The model under review builds one solid part; all positions refer to its coordinate system, in mm. A direction names the side the tool comes from. Give positions to 0.01 mm unless a question says otherwise; leave off trailing zeros. Loops run counter-clockwise (first coordinate to the right, second up) from the corner with the lowest first, then second, coordinate; pieces in that order, holes last. Notation, with made-up numbers: (-13, 71.5) - (24, 71.5) arc R26 ccw to (24, 87.5) - close; hole circle Ø5 at (-26, 57). An arc over 180 degrees is marked (long way). Return JSON: item names as keys, results as strings. Group by question number.
```python
from build123d import *

# Parameters (mm, degrees)
BOSS_EXTRUDE1_DEPTH = 24
SKETCH3_R           = 1.1
BOSS_EXTRUDE6_DEPTH = 2
SHELL1_START        = 2.5
SHELL1_OUTLINE_W    = 40
SHELL1_OUTLINE_H    = 21
SHELL1_DEPTH        = 10.5
SHELL1_START_2      = 12.5
SHELL1_2_DEPTH      = 0.5
SHELL1_START_3      = 1.5
SHELL1_3_DEPTH      = 21
CUT_EXTRUDE1_START  = 16.6
SKETCH5_W           = 3.5
SKETCH5_H           = 5
CUT_EXTRUDE1_DEPTH  = 4.9
FILLET1_R           = 0.5


with BuildPart() as part:
    # Sketch1 → Boss-Extrude1 (new body)
    with BuildSketch(Plane.XY):
        with BuildLine():
            Line((-21.5, 13), (21.5, 13))
            Line((21.5, 13), (21.5, 2.5))
            ThreePointArc((21.5, 2.5), (20.767766953, 0.732233047), (19, 0))
            Line((19, 0), (-19, 0))
            ThreePointArc((-19, 0), (-20.767766953, 0.732233047), (-21.5, 2.5))
            Line((-21.5, 2.5), (-21.5, 13))
        make_face()
    extrude(amount=BOSS_EXTRUDE1_DEPTH)

    # Sketch3 → Boss-Extrude6 (add)
    # profile 1 of 4: a face of its own
    with BuildSketch(Plane(origin=(0, 13, 0), x_dir=(-1, 0, 0), z_dir=(0, 1, 0))):
        with BuildLine():
            Line((16.6, 0), (10.4, 0))
            Line((10.4, 0), (10.4, -2.5))
            ThreePointArc((10.4, -2.5), (13.5, -5.6), (16.6, -2.5))
            Line((16.6, -2.5), (16.6, 0))
        make_face()
        with Locations(Location((13.5, -2.5, 0), (0, 0, 90))):
            Circle(SKETCH3_R, mode=Mode.SUBTRACT)
    # profile 2 of 4: a face of its own
    with BuildSketch(Plane(origin=(0, 13, 0), x_dir=(-1, 0, 0), z_dir=(0, 1, 0))):
        with BuildLine():
            Line((-10.4, 0), (-16.6, 0))
            Line((-16.6, 0), (-16.6, -2.5))
            ThreePointArc((-16.6, -2.5), (-13.5, -5.6), (-10.4, -2.5))
            Line((-10.4, -2.5), (-10.4, 0))
        make_face()
        with Locations(Location((-13.5, -2.5, 0), (0, 0, 90))):
            Circle(SKETCH3_R, mode=Mode.SUBTRACT)
    # profile 3 of 4: a face of its own
    with BuildSketch(Plane(origin=(0, 13, 0), x_dir=(-1, 0, 0), z_dir=(0, 1, 0))):
        with BuildLine():
            Line((-16.6, 26.5), (-16.6, 24))
            Line((-16.6, 24), (-10.4, 24))
            Line((-10.4, 24), (-10.4, 26.5))
            ThreePointArc((-10.4, 26.5), (-13.5, 29.6), (-16.6, 26.5))
        make_face()
        with Locations(Location((-13.5, 26.5, 0), (0, 0, 90))):
            Circle(SKETCH3_R, mode=Mode.SUBTRACT)
    # profile 4 of 4: a face of its own
    with BuildSketch(Plane(origin=(0, 13, 0), x_dir=(-1, 0, 0), z_dir=(0, 1, 0))):
        with BuildLine():
            Line((10.4, 26.5), (10.4, 24))
            Line((10.4, 24), (16.6, 24))
            Line((16.6, 24), (16.6, 26.5))
            ThreePointArc((16.6, 26.5), (13.5, 29.6), (10.4, 26.5))
        make_face()
        with Locations(Location((13.5, 26.5, 0), (0, 0, 90))):
            Circle(SKETCH3_R, mode=Mode.SUBTRACT)
    extrude(amount=-BOSS_EXTRUDE6_DEPTH)

    # Shell1: read off the stored shape, not the designer's step
    # Shell1 outline → Shell1 (cut)
    with BuildSketch(Plane(origin=(0, 0, 0), x_dir=(1, 0, 0), z_dir=(0, 1, 0)).offset(SHELL1_START)):
        with Locations((0, -12)):
            Rectangle(SHELL1_OUTLINE_W, SHELL1_OUTLINE_H)
    extrude(amount=SHELL1_DEPTH, mode=Mode.SUBTRACT)

    # Shell1 2 outline → Shell1 2 (cut)
    with BuildSketch(Plane(origin=(0, 0, 0), x_dir=(1, 0, 0), z_dir=(0, 1, 0)).offset(SHELL1_START_2)):
        with BuildLine():
            Line((-15.1, 0.450609847), (-15.1, -1.5))
            Line((-15.1, -1.5), (-11.9, -1.5))
            Line((-11.9, -1.5), (-11.9, 0.450609847))
            ThreePointArc((-11.9, 0.450609847), (-13.5, -0.1), (-15.1, 0.450609847))
        make_face()
        with BuildLine():
            Line((-11.9, -22.5), (-15.1, -22.5))
            Line((-15.1, -22.5), (-15.1, -24.450609847))
            ThreePointArc((-15.1, -24.450609847), (-13.5, -23.9), (-11.9, -24.450609847))
            Line((-11.9, -24.450609847), (-11.9, -22.5))
        make_face()
        with BuildLine():
            Line((11.9, 0.450609847), (11.9, -1.5))
            Line((11.9, -1.5), (15.1, -1.5))
            Line((15.1, -1.5), (15.1, 0.450609847))
            ThreePointArc((15.1, 0.450609847), (13.5, -0.1), (11.9, 0.450609847))
        make_face()
        with BuildLine():
            Line((15.1, -22.5), (11.9, -22.5))
            Line((11.9, -22.5), (11.9, -24.450609847))
            ThreePointArc((11.9, -24.450609847), (13.5, -23.9), (15.1, -24.450609847))
            Line((15.1, -24.450609847), (15.1, -22.5))
        make_face()
    extrude(amount=SHELL1_2_DEPTH, mode=Mode.SUBTRACT)

    # Shell1 3 outline → Shell1 3 (cut)
    with BuildSketch(Plane.XY.offset(SHELL1_START_3)):
        with BuildLine():
            ThreePointArc((19, 1.5), (19.707106781, 1.792893219), (20, 2.5))
            Line((20, 2.5), (-20, 2.5))
            ThreePointArc((-20, 2.5), (-19.707106781, 1.792893219), (-19, 1.5))
            Line((-19, 1.5), (19, 1.5))
        make_face()
    extrude(amount=SHELL1_3_DEPTH, mode=Mode.SUBTRACT)

    # Sketch5 → Cut-Extrude1 (cut)
    with BuildSketch(Plane(origin=(0, 0, 0), x_dir=(0, 0, -1), z_dir=(1, 0, 0)).offset(CUT_EXTRUDE1_START)):
        with Locations((-22.25, 10.5)):
            Rectangle(SKETCH5_W, SKETCH5_H)
    extrude(amount=CUT_EXTRUDE1_DEPTH, mode=Mode.SUBTRACT)

    # Fillet1
    fillet1_edges = [part.edges().sort_by_distance(p)[0] for p in [
        (-10.4, 12, 24),
        (-16.6, 12, 24),
        (10.4, 12, 24),
        (10.4, 12, 0),
        (16.6, 12, 0),
        (-10.4, 12, 0),
        (-16.6, 12, 0),
        (13.5, 11, 0),
        (-13.5, 11, 0),
        (13.5, 11, 24),
        (-13.5, 11, 24),
    ]]
    fillet(fillet1_edges, radius=FILLET1_R)


solid = part.part
```
1) Tool access review of faces 1 (the face through (-14, 11, -4)), 2 (the face through (-20, 8, 12)), 3 (the face through (10.4, 12, 25)), 4 (the face through (-16.6, 12, -2)): name each direction out of +Z, -Z, +X, -X, +Y, -Y from which nothing blocks a thin tool from reaching the whole face with its end or side.
2) For pin 1 Ø1 at (y, z) = (12.5, 25.5) entering from -X; pin 2 Ø0.6 at (x, z) = (13, 23.5) entering from +Y; pin 3 Ø3 at (x, y) = (-4, 7.5) entering from +Z, all flat-tipped, find the tip position at first contact; note any pin that passes through.
3) We need section C-C, the plane z = 5.5. Write out the cut boundary in (x, y), plus the area to 3 significant figures.
4) Draft analysis for pull direction Z (two halves, no side actions). For faces 5 (the face through (13, 12.5, 23)), 6 (the face through (-10.4, 12, 26)), 7 (the face through (13.6, 12, -5.6)), 8 (the face through (13.4, 12, 29.6)), state which applies: +Z half, -Z half, draft (parallel to the pull), parting line (faces both ways), or undercut.
5) We need section A-A, the plane y = 4.25. Write out the cut boundary in (x, z).
6) We need section B-B, the plane x = -13.5. Write out the cut boundary in (y, z).
7) To check wall thickness, follow line 1 (X direction, y = 12.5, z = 26.5); line 2 (Z direction, x = 0, y = 10.5); line 3 (X direction, y = 11.25, z = 8). State the ranges of each line that lie inside material, in increasing order.
8) We need section D-D, the plane x = -4. Write out the cut boundary in (y, z), plus the area to 3 significant figures.
Findings:
{
 "1": {"face 1": "-Z, +X, -X, -Y", "face 2": "+Y", "face 3": "+Z, +Y, -Y", "face 4": "-Z, -X, +Y, -Y"},
 "2": {"pin 1": "stops at x = -16.6", "pin 2": "stops at y = 12.5", "pin 3": "stops at z = 24"},
 "3": {"outline": "(-21.5, 2.5) arc R2.5 ccw to (-19, 0) - (19, 0) arc R2.5 ccw to (21.5, 2.5) - (21.5, 13) - (20, 13) - (20, 2.5) arc R1 cw to (19, 1.5) - (-19, 1.5) arc R1 cw to (-20, 2.5) - (-20, 13) - (-21.5, 13) - close", "area": "96.7 mm^2"},
 "4": {"face 5": "undercut", "face 6": "draft", "face 7": "-Z half", "face 8": "+Z half"},
 "5": {"outline": "(-21.5, 0) - (21.5, 0) - (21.5, 24) - (-21.5, 24) - close; hole (-20, 1.5) - (20, 1.5) - (20, 22.5) - (-20, 22.5) - close"},
 "6": {"outline": "(0, 0) - (10.5, 0) arc R0.5 cw to (11, -0.5) - (11, -1.4) - (13, -1.4) - (13, 0.1) - (12.5, 0.1) - (12.5, 1.5) - (1.5, 1.5) - (1.5, 22.5) - (12.5, 22.5) - (12.5, 23.9) - (13, 23.9) - (13, 25.4) - (11, 25.4) - (11, 24.5) arc R0.5 cw to (10.5, 24) - (0, 24) - close; (11, -5.6) - (13, -5.6) - (13, -3.6) - (11, -3.6) - close; (11, 27.6) - (13, 27.6) - (13, 29.6) - (11, 29.6) - close"},
 "7": {"line 1": "x = -16.6 to -14.6, -12.4 to -10.4, 10.4 to 12.4, 14.6 to 16.6", "line 2": "z = 0 to 1.5, 22.5 to 24", "line 3": "x = -21.5 to -20, 20 to 21.5"},
 "8": {"outline": "(0, 0) - (13, 0) - (13, 1.5) - (1.5, 1.5) - (1.5, 22.5) - (13, 22.5) - (13, 24) - (0, 24) - close", "area": "70.5 mm^2"}
}
